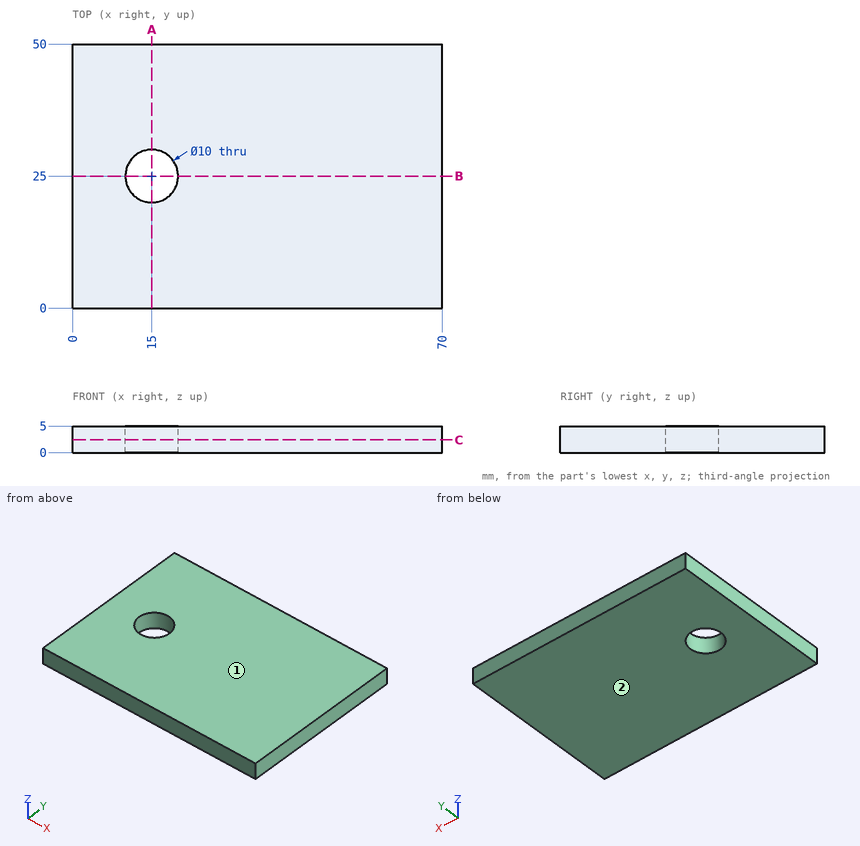
Here's the drawing with two shaded views (mm, measured from the low corner). I have some questions. Round coordinates to 2 decimals unless told otherwise and drop trailing zeros. Order: outer loops, then holes, each group sorted by start corner. A loop starts at its lowest first (then second) coordinate and runs counter-clockwise, first axis right, second up. Notation, with made-up numbers: M 81.5,20 L 132.5,20 A30 cw 132.5,57 Z; hole C 58,-21 d8. An arc over 180 degrees is marked long. Use CSV: the item, a comma, the result in double quotes.
1) I need wall thicknesses on line 1 along Y through (x, z) = (15, 2.7); line 2 along X through (y, z) = (24.5, 4.5); line 3 along Y through (x, z) = (19.5, 4.7). Which ranges of each line are inside material? Lowest first, please. Write a range as [from, to].
Taken from the geometry:
line 1,"[0, 20], [30, 50]"
line 2,"[0, 10.03], [19.97, 70]"
line 3,"[0, 22.82], [27.18, 50]"
2) If we mould it in two halves opening along Z, with no side actions, what happens to the marked faces 1 and 2? For each: pulls with the +Z half, pulls with the -Z half, needs draft (parallel to the pull), parting line crosses it, or undercut.
Taken from the geometry:
face 1,"pulls with the +Z half"
face 2,"pulls with the -Z half"
3) I want a section at A-A (x = 15). List the corners of the cut face in (y, z) for me.
Taken from the geometry:
outline,"M 0,0 L 20,0 L 20,5 L 0,5 Z; M 30,0 L 50,0 L 50,5 L 30,5 Z"
4) I want a section at C-C (z = 2.4). List the corners of the cut face in (x, y) for me.
Taken from the geometry:
outline,"M 0,0 L 70,0 L 70,50 L 0,50 Z; hole C 15,25 d10"
5) I want a section at B-B (y = 25). List the corners of the cut face in (x, z) for me, then the cut area to 3 significant figures.
Taken from the geometry:
outline,"M 0,0 L 10,0 L 10,5 L 0,5 Z; M 20,0 L 70,0 L 70,5 L 20,5 Z"
area,"300 mm^2"
6) I'm going to push a flat-ended pin straight in: P1, Ø8, axis at x = 15, y = 25, coming from the +Z side. Where does the tip first touch, or does it pass through?
Taken from the geometry:
P1,"through"
